CAD build for the part. Positions are in the model's coordinates, mm. A direction names the side the tool comes from. Coordinates: 2 decimals unless noted, no trailing zeros. Write each loop counter-clockwise with the first axis right and the second up, starting at its lowest first coordinate (ties: lowest second). Pieces come first, ordered by that corner, then holes.
```python
from build123d import *

# Parameters (mm, degrees)
F1_DEPTH = 10
F2_R     = 1.25
F3_DEPTH = 25


with BuildPart() as f1:
    # F0 (on Front) → F1 (new body)
    with BuildSketch(Plane.XZ):
        Polygon((-3, 0), (0, 0), (2, 5), (0, 5), (0, 6.4), (1.5, 6.4), (1.5, 7.9), (26.5, 7.9), (26.5, 9.9), (2.062178, 9.9), (-1.955755, 7.580245), (-3, 6), (-3, 5), (-2, 5), align=None)
    extrude(amount=F1_DEPTH)

    # F2 (on face) → F3 (cut)
    with BuildSketch(Plane.XY.offset(9.9)):
        with Locations((23, -5)):
            Circle(F2_R)
    extrude(amount=-F3_DEPTH, mode=Mode.SUBTRACT)


solid = f1.part
```
Item 1: Two-plate mould, pull along Z, no slides. Class faces 1 (the flat face through (9.5, 0, 8.3)), 2 (the flat face through (1, -4.9, 2.5)), 3 (the flat face through (1, -5, 5)): +Z half, -Z half, draft (parallel to the pull), parting line (faces both ways), or undercut.
Item 2: Which spindle directions (+Z, -Z, +X, -X, +Y, -Y) get a long thin tool onto all of the face, cutting with end or side? Do faces 4 (the flat face through (-2, -5, 0)), 5 (the flat face through (0, -5, 6)), 6 (the flat face through (-2.5, -4.9, 2.5)). Say none if no direction does.
Item 3: Saw through at D-D, the plane y = -1.75. Write the cut outline in (x, z).
Item 4: Saw through at C-C, the plane z = 8.75. Write the cut outline in (x, y).
Item 5: Flat gauge pins, fed straight in: pin 1 Ø1 at (x, z) = (1.5, 2.5) entering from -Y; pin 2 Ø1 at (x, y) = (1.5, -6.5) entering from +Z; pin 3 Ø5 at (x, y) = (20, -7) entering from -Z. Where does each tip first touch, or does it go through?
Item 6: Saw through at A-A, the plane x = 23. Write the cut outline in (y, z), and give its area (3 significant figures).
Item 7: Saw through at B-B, the plane y = -5. Write the cut outline in (x, z), and give its area (3 significant figures).
Item 8: Wall check: line 1 along Y through (x, z) = (23, 8.45); line 2 along Z through (x, y) = (4, -1); line 3 along Y through (x, z) = (22, 9.5). Give the ranges that are in metal, low to high.
Working result:
1. face 1: draft
1. face 2: -Z half
1. face 3: undercut
2. face 4: -Z, +X, -X, +Y, -Y
2. face 5: +X, +Y, -Y
2. face 6: -X, +Y, -Y
3. outline: (-3, 0) - (0, 0) - (2, 5) - (0, 5) - (0, 6.4) - (1.5, 6.4) - (1.5, 7.9) - (26.5, 7.9) - (26.5, 9.9) - (2.06, 9.9) - (-1.96, 7.58) - (-3, 6) - (-3, 5) - (-2, 5) - close
4. outline: (0.07, -10) - (26.5, -10) - (26.5, 0) - (0.07, 0) - close; hole circle Ø2.5 at (23, -5)
5. pin 1: stops at y = -10
5. pin 2: stops at z = 9.86
5. pin 3: stops at z = 7.9
6. outline: (-10, 7.9) - (-6.25, 7.9) - (-6.25, 9.9) - (-10, 9.9) - close; (-3.75, 7.9) - (0, 7.9) - (0, 9.9) - (-3.75, 9.9) - close
6. area: 15.0 mm2
7. outline: (-3, 0) - (0, 0) - (2, 5) - (0, 5) - (0, 6.4) - (1.5, 6.4) - (1.5, 7.9) - (21.75, 7.9) - (21.75, 9.9) - (2.06, 9.9) - (-1.96, 7.58) - (-3, 6) - (-3, 5) - (-2, 5) - close; (24.25, 7.9) - (26.5, 7.9) - (26.5, 9.9) - (24.25, 9.9) - close
7. area: 74.5 mm2
8. line 1: y = -10 to -6.25, -3.75 to 0
8. line 2: z = 7.9 to 9.9
8. line 3: y = -10 to -5.75, -4.25 to 0
